Autodesk Inventor part; units mm, degrees
ref_plane "YZ Plane" through (0, 0, 0) normal (1, 0, 0) x (0, 1, 0)
ref_plane "XZ Plane" through (0, 0, 0) normal (0, 1, 0) x (-1, 0, 0)
ref_plane "XY Plane" through (0, 0, 0) normal (0, 0, 1) x (1, 0, 0)
sketch "Sketch1" plane through (0, 0, 0) normal (0, 1, 0) x (-1, 0, 0)
  circle A0 centre (0, 0) radius 2.7
  circle A1 centre (0, 0) radius 5.5
  dimension "d0" = 5.4
  dimension "d1" = 11
extrude "Extrusion1" add sketch "Sketch1" along normal blind 5.4
sketch "Sketch2" plane through (0, 5.4, 0) normal (0, 1, 0) x (1, 0, 0)
  circle A0 centre (0, 0) radius 7.3
  dimension "d4" = 14.6
extrude "Extrusion2" add sketch "Sketch2" along normal blind 3
sketch "Sketch3" plane through (0, 8.4, 0) normal (0, 1, 0) x (1, 0, 0)
  arc A0 (3.5, 32) -> (-3.5, 32) centre (0, 32) ccw
  circle A1 centre (0, 0) radius 7.3
  line L0 (-7.3, 0) -> (-3.5, 32)
  line L1 (7.3, 0) -> (3.5, 32)
  dimension "d7" = 7
  dimension "d8" = 32
extrude "Extrusion3" add sketch "Sketch3" against normal blind 3 contours L1 A1 L0 A0 | L1 A1 L0
sketch "Sketch5" plane through (0, 8.4, 0) normal (0, 1, 0) x (1, 0, 0)
  point P0 (0, 0)
  point P1 (0, 28.89)
  dimension "d18" = 28.89
hole "Hole2" at (0, 8.4, -28.89) direction (0, -1, 0) diameter 3 end through all
properties part number "big_servo_arm"
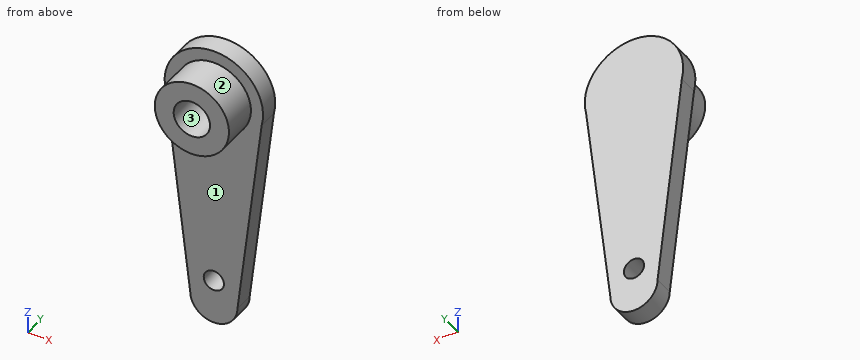
Design review of the part built by this model. Coordinates are the model's own, in mm. Face numbers are marked on the shaded views. Coordinates: 2 decimals unless noted, no trailing zeros. Order: outer loops, then holes, each group sorted by start corner. A loop starts at its lowest first (then second) coordinate and runs counter-clockwise, first axis right, second up.
Item 1: Take a section at D-D, the plane z = -28.89. Write out the cut boundary in (x, y).
Item 2: Take a section at B-B, the plane y = 7.25. Write out the cut boundary in (x, z), then the cut area to 3 significant figures.
Item 3: Take a section at C-C, the plane z = 0. Write out the cut boundary in (x, y), then the cut area to 3 significant figures.
Item 4: For pin 1 Ø1.5 at (y, z) = (4, 0) entering from +X; pin 2 Ø2 at (x, z) = (-1.5, -21.5) entering from -Y; pin 3 Ø4 at (y, z) = (6.5, -16.5) entering from +X, all flat-tipped, find the tip position at first contact; note any pin that passes through.
Item 5: For line 1 (Z direction, x = 0, y = 7.1); line 2 (Y direction, x = 1.25, z = -25.5); line 3 (Z direction, x = -2, y = 3.25), list the stretches that pass through material, from the lowest coordinate up.
Item 6: Take a section at A-A, the plane x = 0. Write out the cut boundary in (y, z), then the cut area to 3 significant figures.
Item 7: The part is to be moulded in two halves that separate along Z. For the marked faces 1, 2 and 3, say which applies: pulls with the +Z half, pulls with the -Z half, needs draft (parallel to the pull), parting line crosses it, or undercut.
The answers:
1. outline: (-3.87, 5.4) - (-1.5, 5.4) - (-1.5, 8.4) - (-3.87, 8.4) - close; (1.5, 5.4) - (3.87, 5.4) - (3.87, 8.4) - (1.5, 8.4) - close
2. outline: (-7.1, -1.71) - (-3.5, -32) arc R3.5 ccw to (3.5, -32) - (7.1, -1.71) arc R7.3 ccw (long way) to start; hole circle Ø3 at (0, -28.89)
2. area: 442 mm2
3. outline: (-7.3, 5.4) - (-5.5, 5.4) - (-5.5, 0) - (-2.7, 0) - (-2.7, 5.4) - (2.7, 5.4) - (2.7, 0) - (5.5, 0) - (5.5, 5.4) - (7.3, 5.4) - (7.3, 8.4) - (-7.3, 8.4) - close
3. area: 74.0 mm2
4. pin 1: stops at x = 5.5
4. pin 2: stops at y = 5.4
4. pin 3: stops at x = 5.58
5. line 1: z = -35.5 to -30.39, -27.39 to 7.3
5. line 2: y = 5.4 to 8.4
5. line 3: z = -5.12 to -1.81, 1.81 to 5.12
6. outline: (0, -5.5) - (5.4, -5.5) - (5.4, -27.39) - (8.4, -27.39) - (8.4, 7.3) - (5.4, 7.3) - (5.4, 5.5) - (0, 5.5) - (0, 2.7) - (5.4, 2.7) - (5.4, -2.7) - (0, -2.7) - close; (5.4, -35.5) - (8.4, -35.5) - (8.4, -30.39) - (5.4, -30.39) - close
6. area: 150 mm2
7. face 1: needs draft
7. face 2: parting line crosses it
7. face 3: undercut
